from build123d import *

# Parameters (mm, degrees)
SKETCH1_R           = 1.5
SKETCH1_W           = 50
SKETCH1_H           = 70
BOSS_EXTRUDE1_DEPTH = 2.5
SKETCH2_W           = 3.429676715
SKETCH2_H           = 22.352
BOSS_EXTRUDE2_DEPTH = 1


with BuildPart() as part:
    # Sketch1 → Boss-Extrude1 (new body)
    with BuildSketch(Plane.XY):
        Polygon((100, 100), (-100, 100), (-100, -97.5), (-60, -97.5), (-60, -100), (-20, -100), (-20, -97.5), (20, -97.5), (20, -100), (60, -100), (60, -97.5), (100, -97.5), align=None)
        with Locations((-90, -60)):
            Circle(SKETCH1_R, mode=Mode.SUBTRACT)
        with Locations((-90, 0)):
            Circle(SKETCH1_R, mode=Mode.SUBTRACT)
        with Locations((0, -50)):
            Rectangle(SKETCH1_W, SKETCH1_H, mode=Mode.SUBTRACT)
        with Locations((90, -60)):
            Circle(SKETCH1_R, mode=Mode.SUBTRACT)
        with Locations((90, 0)):
            Circle(SKETCH1_R, mode=Mode.SUBTRACT)
        with Locations((-90, 60)):
            Circle(SKETCH1_R, mode=Mode.SUBTRACT)
        with Locations((90, 60)):
            Circle(SKETCH1_R, mode=Mode.SUBTRACT)
    extrude(amount=BOSS_EXTRUDE1_DEPTH)

    # Sketch2 → Boss-Extrude2 (add)
    with BuildSketch(Plane.XY.offset(2.5)):
        Polygon((-13.574972078, -2.206402508), (-22.362641896, -2.206402508), (-22.362641896, 5.396315859), (-14.538404318, 5.396315859), (-14.538404318, 8.0657162), (-22.362641896, 8.0657162), (-22.362641896, 14.587158479), (-14.071285656, 14.587158479), (-14.071285656, 17.256562946), (-25.792318612, 17.256562946), (-25.792318612, -4.875802849), (-13.574972078, -4.875802849), align=None)
        with BuildLine():
            Line((-1.32204553, 6.603648154), (4.762112339, 17.501539559))
            Line((4.762112339, 17.501539559), (0.995728896, 17.501539559))
            Line((0.995728896, 17.501539559), (-1.437934251, 12.6228991))
            add(Edge.make_bspline(
                [(-1.437934251, 12.6228991), (-1.596718144, 12.303861859), (-1.904219722, 11.686012946), (-2.342902996, 10.763464709), (-2.769861176, 9.837525479), (-3.03923337, 9.20683016), (-3.17843881, 8.880901126)],
                knots=[0, 0, 0, 0, 1.03599958, 2.006321307, 2.969712076, 4, 4, 4, 4], degree=3))
            Line((-3.17843881, 8.880901126), (-3.234209432, 8.882782007))
            add(Edge.make_bspline(
                [(-3.234209432, 8.882782007), (-3.377496248, 9.189095467), (-3.661154937, 9.795490923), (-4.089483987, 10.709635801), (-4.532333468, 11.641980958), (-4.843108785, 12.270176419), (-5.003092207, 12.593563942)],
                knots=[0, 0, 0, 0, 0.987131341, 1.954181056, 2.946836831, 4, 4, 4, 4], degree=3))
            Line((-5.003092207, 12.593563942), (-7.46414776, 17.501539559))
            Line((-7.46414776, 17.501539559), (-11.259503382, 17.501539559))
            Line((-11.259503382, 17.501539559), (-5.349178596, 6.51598916))
            Line((-5.349178596, 6.51598916), (-11.490752858, -4.850460441))
            Line((-11.490752858, -4.850460441), (-7.753869563, -4.850460441))
            Line((-7.753869563, -4.850460441), (-5.465067317, -0.087655081))
            add(Edge.make_bspline(
                [(-5.465067317, -0.087655081), (-5.364335932, 0.114078616), (-5.167684585, 0.507910222), (-4.884459094, 1.085166952), (-4.624500068, 1.634448669), (-4.297310404, 2.31859573), (-3.914960495, 3.148810565), (-3.634210423, 3.815857985), (-3.495218913, 4.146094507)],
                knots=[0, 0, 0, 0, 0.869006123, 1.696504258, 2.478000857, 3.2109747, 4.619231574, 6, 6, 6, 6], degree=3))
            Line((-3.495218913, 4.146094507), (-3.408042514, 4.149196312))
            add(Edge.make_bspline(
                [(-3.408042514, 4.149196312), (-3.255611823, 3.817980032), (-2.94839099, 3.150420628), (-2.536943481, 2.319070478), (-2.189297936, 1.63260853), (-1.901799923, 1.085781735), (-1.594451142, 0.505813053), (-1.376920295, 0.112098507), (-1.265086983, -0.090311414)],
                knots=[0, 0, 0, 0, 1.381153135, 2.783684921, 3.513572612, 4.296050064, 5.123993829, 6, 6, 6, 6], degree=3))
            Line((-1.265086983, -0.090311414), (1.169561978, -4.850460441))
            Line((1.169561978, -4.850460441), (4.964917601, -4.850460441))
            Line((4.964917601, -4.850460441), (-1.32204553, 6.603648154))
        make_face()
        with Locations((9.442078464, 6.325539559)):
            Rectangle(SKETCH2_W, SKETCH2_H)
        Polygon((29.36462049, 17.50216652), (13.877443327, 17.50216652), (13.877443327, 14.611869802), (19.891596092, 14.611869802), (19.891596092, -4.831944479), (23.321272808, -4.831944479), (23.321272808, 14.611869802), (29.36462049, 14.611869802), align=None)
    extrude(amount=BOSS_EXTRUDE2_DEPTH)


solid = part.part
Geometry: final body of the model. Coordinates: model frame, mm. A direction names the side the tool comes from. Give positions to 0.01 mm unless a question says otherwise; leave off trailing zeros. Write each loop counter-clockwise with the first axis right and the second up, starting at its lowest first coordinate (ties: lowest second). Pieces come first, ordered by that corner, then holes.
(1) Access query for faces 4 (the flat face through (-21, 6, 3.5)), 5 (the flat face through (1.865, 0.796, 2.993)). Directions: +Z, -Z, +X, -X, +Y, -Y. A direction counts if a zero-diameter tool reaches every point of the face in a straight line with its end or side. Return the directions, or none.
(2) First-contact query: P1, Ø0.5, axis at x = -22, z = 3, coming from the -Y side; P2, Ø1.2, axis at y = -99, z = 1.5, coming from the -X side; P3, Ø1.1, axis at x = -16, z = 3, coming from the -Y side. Flat tips, straight axial feed; report the tip coordinate or a pass-through.
(3) Mould query, pull axis X, two halves, no side actions, for faces 1 (the flat face through (-1, 1, 0)), 2 (the flat face through (-8.35, 12.09, 2.99)), 3 (the flat face through (1.68, 11.98, 2.99)). Classes: released by +X, released by -X, zero draft, split by the parting line, or undercut.
(4) Cut plane A-A, the plane z = 1.8. Return loops of the section in (x, y), then the cut area to 3 significant figures.
(5) Cut plane B-B, the plane y = 64. Return loops of the section in (x, z).
(6) Ray query, line 1 (Y direction, x = -90, z = 0.95); line 2 (X direction, y = -65.5, z = 2.4); line 3 (X direction, y = -61, z = 1.1). Return the intervals inside material, ascending.
Values follow:
1. face 4: +Z, +X, -X, +Y, -Y
1. face 5: +Z
2. P1: stops at y = -4.88
2. P2: stops at x = -60
2. P3: stops at y = -97.5
3. face 1: zero draft
3. face 2: undercut
3. face 3: undercut
4. outline: (-100, -97.5) - (-60, -97.5) - (-60, -100) - (-20, -100) - (-20, -97.5) - (20, -97.5) - (20, -100) - (60, -100) - (60, -97.5) - (100, -97.5) - (100, 100) - (-100, 100) - close; hole circle Ø3 at (-90, -60); hole circle Ø3 at (-90, 0); hole circle Ø3 at (-90, 60); hole (-25, -85) - (25, -85) - (25, -15) - (-25, -15) - close; hole circle Ø3 at (90, -60); hole circle Ø3 at (90, 0); hole circle Ø3 at (90, 60)
4. area: 36,200 mm2
5. outline: (-100, 0) - (100, 0) - (100, 2.5) - (-100, 2.5) - close
6. line 1: y = -97.5 to -61.5, -58.5 to -1.5, 1.5 to 58.5, 61.5 to 100
6. line 2: x = -100 to -25, 25 to 100
6. line 3: x = -100 to -91.12, -88.88 to -25, 25 to 88.88, 91.12 to 100
